Check sheet for the drawn part. Datum: minimum x, y, z corner. Units: mm. Coordinates: 2 decimals unless noted, no trailing zeros. Order: outer loops, then holes, each group sorted by start corner. A loop starts at its lowest first (then second) coordinate and runs counter-clockwise, first axis right, second up. Notation, with made-up numbers: (-26.75, -11) - (-15.75, -11) arc R21 ccw to (-15.75, 18) - close; hole circle Ø7 at (-33, 60). An arc over 180 degrees is marked (long way). Answer as CSV lines item,"result". Start each with the question number.
1. Section check C-C (z = 247). Record the cut outline in (x, y), and give its area (3 significant figures).
2. Section check A-A (z = 350). Record the cut outline in (x, y), and give its area (3 significant figures).
3. Go/stop test with flat-tipped pins: pin 1 (6 mm diameter, centred on x = 126, z = 148.5, fed in from -Y); pin 2 (8 mm diameter, centred on x = 196.5, y = 13.5, fed in from -Z); pin 3 (6 mm diameter, centred on y = 8.02, z = 350, fed in from -X); pin 4 (5 mm diameter, centred on x = 195.5, y = 13.5, fed in from +Z). Record where each tip stops, or that it passes through.
4. Material ranges on L1, parallel to Y at x = 105, z = 170.5; L2, parallel to X at y = 14.75, z = 353.5, recorded low to high. Write a range as [from, to].
5. Section check B-B (x = 173). Record the cut outline in (y, z), and give its area (3 significant figures).
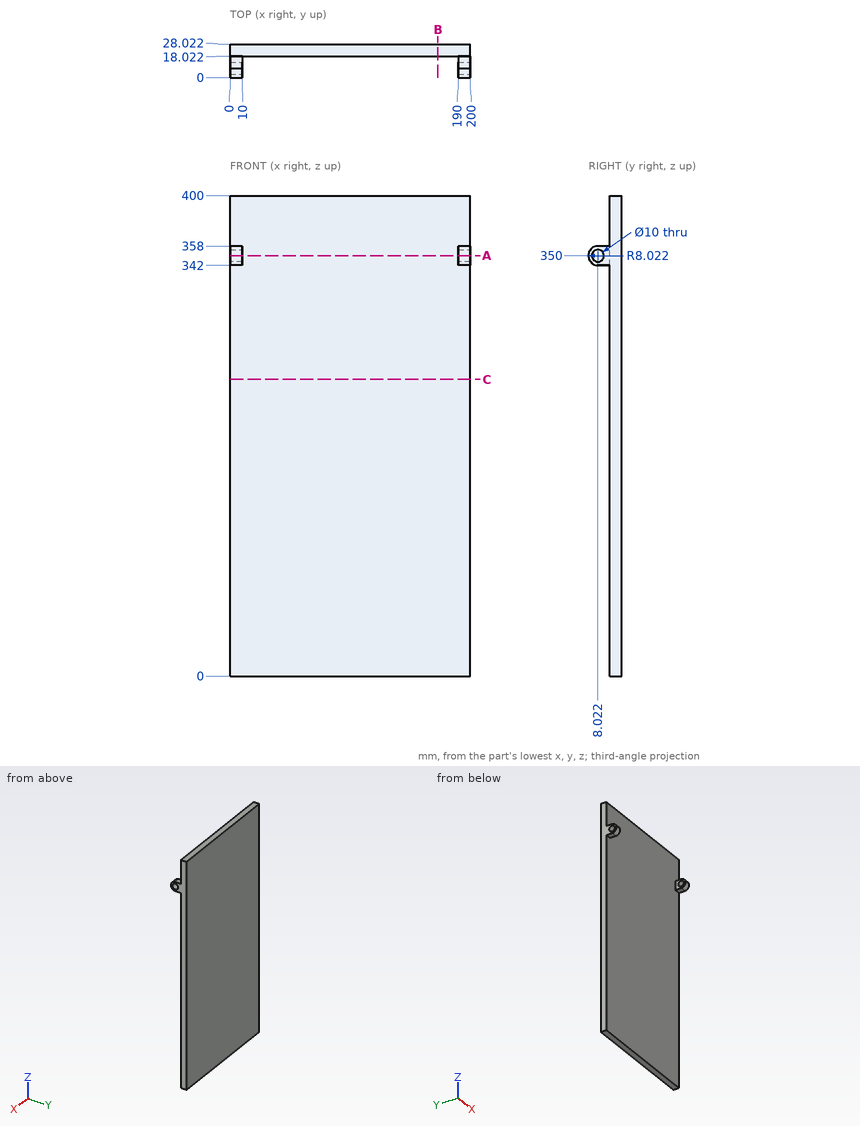
Evaluation:
1,outline,"(0, 18.02) - (200, 18.02) - (200, 28.02) - (0, 28.02) - close"
1,area,"2,000 mm²"
2,outline,"(0, 0) - (10, 0) - (10, 3.02) - (0, 3.02) - close; (0, 13.02) - (10, 13.02) - (10, 18.02) - (190, 18.02) - (190, 13.02) - (200, 13.02) - (200, 28.02) - (0, 28.02) - close; (190, 0) - (200, 0) - (200, 3.02) - (190, 3.02) - close"
2,area,"2,160 mm²"
3,pin 1,"stops at y = 18.02"
3,pin 2,"stops at z = 342"
3,pin 3,"passes through"
3,pin 4,"stops at z = 358"
4,L1,"y = [18.02, 28.02]"
4,L2,"x = [0, 10], [190, 200]"
5,outline,"(18.02, 0) - (28.02, 0) - (28.02, 400) - (18.02, 400) - close"
5,area,"4,000 mm²"
